```python
from build123d import *

# Parameters (mm, degrees)
F0_W         = 292.1
F0_H         = 558.8
F1_DEPTH     = 19.05
F3_W         = 19.05
F3_H         = 558.8
F4_DEPTH     = 6.35
F5_T1_DEPTH  = 320.675
F5_T3_DEPTH  = 520.7
F5_T5_DEPTH  = 47.625
F5_S9_W      = 19.05
F5_S9_H      = 19.05
F5_T10_DEPTH = 19.05
F5_S15_W     = 19.05
F5_S15_H     = 19.05
F5_T16_DEPTH = 19.05
F6_W         = 19.05
F6_H         = 558.8
F7_DEPTH     = 19.05


# Not quite as in the source:
# - a fillet or chamfer that OpenCascade refuses, or shapes differently, is made with other operations: its cross-section is extruded or revolved along the edge and cut away or added


with BuildPart() as f1:
    # F0 (on Front) → F1 (new body)
    with BuildSketch(Plane.XZ):
        Rectangle(F0_W, F0_H)
    extrude(amount=-F1_DEPTH)

    # F3 (on face) → F4 (cut)
    with BuildSketch(Plane(origin=(0, 19.05, 0), x_dir=(-1, 0, 0), z_dir=(0, 1, 0))):
        with Locations((-111.125, 0)):
            Rectangle(F3_W, F3_H)
    extrude(amount=-F4_DEPTH, mode=Mode.SUBTRACT)

    # F5: fillet of radius 19.05 on 5 edges, made by hand

    # F5_s2 → F5_t1 (cut)
    with BuildSketch(Plane.YZ.offset(-193.675)):
        with BuildLine():
            ThreePointArc((19.05, -279.4), (5.5796158184, -273.8203841816), (0, -260.35))
            Line((0, -260.35), (0, -279.4))
            Line((0, -279.4), (19.05, -279.4))
        make_face()
        with BuildLine():
            ThreePointArc((19.05, 279.4), (5.5796158184, 273.8203841816), (0, 260.35))
            Line((0, 260.35), (0, 279.4))
            Line((0, 279.4), (19.05, 279.4))
        make_face()
    extrude(amount=F5_T1_DEPTH, mode=Mode.SUBTRACT)

    # F5_s4 → F5_t3 (cut)
    with BuildSketch(Plane.XY.offset(-260.35)):
        with BuildLine():
            ThreePointArc((127, 0), (140.4703841816, 5.5796158184), (146.05, 19.05))
            Line((146.05, 19.05), (146.05, 0))
            Line((146.05, 0), (127, 0))
        make_face()
    extrude(amount=F5_T3_DEPTH, mode=Mode.SUBTRACT)

    # F5_s6 → F5_t5 (cut)
    with BuildSketch(Plane.XZ.offset(-66.675)):
        with BuildLine():
            ThreePointArc((127, -279.4), (140.4703841816, -273.8203841816), (146.05, -260.35))
            Line((146.05, -260.35), (146.05, -279.4))
            Line((146.05, -279.4), (127, -279.4))
        make_face()
        with BuildLine():
            ThreePointArc((127, 279.4), (140.4703841816, 273.8203841816), (146.05, 260.35))
            Line((146.05, 260.35), (146.05, 279.4))
            Line((146.05, 279.4), (127, 279.4))
        make_face()
    extrude(amount=F5_T5_DEPTH, mode=Mode.SUBTRACT)


with BuildPart() as f5_tool8:
    # F5_s9 → F5_t10 (new body)
    with BuildSketch(Plane.YZ.offset(127)):
        with Locations((9.525, -269.875)):
            Rectangle(F5_S9_W, F5_S9_H)
    extrude(amount=F5_T10_DEPTH)

    # F5_s11 → F5_t12 (revolve, cut)
    with BuildSketch(Plane(origin=(127, 19.05, -260.35), x_dir=(0, 0.7071067812, 0.7071067812), z_dir=(0, 0.7071067812, -0.7071067812))):
        with BuildLine():
            ThreePointArc((0, -19.05), (19.05, 0), (0, 19.05))
            Line((0, 19.05), (0, -19.05))
        make_face()
    revolve(axis=Axis((127, 19.05, -260.35), (1, 0, 0)), mode=Mode.SUBTRACT)


with BuildPart() as f1_1:
    add(f1.part)

    # F5_t7: cut F5_tool8
    add(f5_tool8.part, mode=Mode.SUBTRACT)


with BuildPart() as f5_tool14:
    # F5_s15 → F5_t16 (new body)
    with BuildSketch(Plane.YZ.offset(127)):
        with Locations((9.525, 269.875)):
            Rectangle(F5_S15_W, F5_S15_H)
    extrude(amount=F5_T16_DEPTH)

    # F5_s17 → F5_t18 (revolve, cut)
    with BuildSketch(Plane(origin=(127, 19.05, 260.35), x_dir=(0, 0.7071067812, -0.7071067812), z_dir=(0, -0.7071067812, -0.7071067812))):
        with BuildLine():
            ThreePointArc((0, -19.05), (19.05, 0), (0, 19.05))
            Line((0, 19.05), (0, -19.05))
        make_face()
    revolve(axis=Axis((127, 19.05, 260.35), (1, 0, 0)), mode=Mode.SUBTRACT)


with BuildPart() as f1_2:
    add(f1_1.part)

    # F5_t13: cut F5_tool14
    add(f5_tool14.part, mode=Mode.SUBTRACT)

    # F6 (on face) → F7 (join)
    with BuildSketch(Plane(origin=(0, 19.05, 0), x_dir=(-1, 0, 0), z_dir=(0, 1, 0))):
        with Locations((114.3, 0)):
            Rectangle(F6_W, F6_H)
    extrude(amount=F7_DEPTH)


solid = f1_2.part
```
Check sheet for the modelled part. Datum: model origin and axes. Units: mm. A direction names the side the tool comes from. Give positions to 0.01 mm unless a question says otherwise; leave off trailing zeros. Order: outer loops, then holes, each group sorted by start corner. A loop starts at its lowest first (then second) coordinate and runs counter-clockwise, first axis right, second up. Notation, with made-up numbers: (34, -32) -> (39, -32) arc R14 ccw to (39, -22) -> close; hole circle Ø11 at (25.5, 83.5). An arc over 180 degrees is marked (long way). Return JSON: item names as keys, results as strings.
1. Cross-section at B-B, the plane y = 27. Record the cut outline in (x, z) (3 decimals), plus the area to 3 significant figures.
From the geometry:
{"outline": "(-123.825, -279.4) -> (-104.775, -279.4) -> (-104.775, 279.4) -> (-123.825, 279.4) -> close", "area": "10,600 mm^2"}
2. Material ranges on probe 1 along X at (y, z) = (18, 118); probe 2 along Y at (x, z) = (4.5, 13.5); probe 3 along X at (y, z) = (33.5, 81) (3 decimals), recorded low to high. Write a range as [from, to].
From the geometry:
{"probe 1": "[-146.05, 101.6], [120.65, 146.02]", "probe 2": "[0, 19.05]", "probe 3": "[-123.825, -104.775]"}
3. Cross-section at C-C, the plane x = 110.5. Record the cut outline in (y, z).
From the geometry:
{"outline": "(0, -260.35) arc R19.05 ccw to (12.7, -278.31) -> (12.7, 278.31) arc R19.05 ccw to (0, 260.35) -> close"}
4. Cross-section at A-A, the plane z = -220. Record the cut outline in (x, y) (3 decimals), plus the area to 3 significant figures.
From the geometry:
{"outline": "(-146.05, 0) -> (127, 0) arc R19.05 ccw to (146.05, 19.05) -> (120.65, 19.05) -> (120.65, 12.7) -> (101.6, 12.7) -> (101.6, 19.05) -> (-104.775, 19.05) -> (-104.775, 38.1) -> (-123.825, 38.1) -> (-123.825, 19.05) -> (-146.05, 19.05) -> close", "area": "5,730 mm^2"}
5. Set-up check for faces 1 (the flat face through (-123.825, 28, -4)), 2 (the flat face through (-3, 19.05, 4)), 3 (the cylindrical face through (-11.44, 5.73, -273.97)), 4 (the flat face through (-146.05, 9, -4)), 5 (the flat face through (111, 12.7, 4)): record each of +Z, -Z, +X, -X, +Y, -Y from which the full face is reachable in a straight line by a thin tool's end or side.
From the geometry:
{"face 1": "+Z, -Z, -X, +Y", "face 2": "+Z, -Z, +X, +Y", "face 3": "-Z, +X, -X, -Y", "face 4": "+Z, -Z, -X, +Y, -Y", "face 5": "+Z, -Z, +Y"}
6. Go/stop test with flat-tipped pins: P1, Ø8, axis at x = 89, y = 20.5, coming from the +Z side; P2, Ø5, axis at x = 77.5, z = -206, coming from the +Y side; P3, Ø5.5, axis at y = 33.5, z = 86.5, coming from the -X side (3 decimals); P4, Ø10, axis at x = 57.5, y = 28.5, coming from the +Z side. Record where each tip stops, or that it passes through.
From the geometry:
{"P1": "z = 279.4", "P2": "y = 19.05", "P3": "x = -123.825", "P4": "through"}
